Verification items for the finished model (mm, model axes). Face numbers are marked on the shaded views. A direction names the side the tool comes from. Round coordinates to 2 decimals unless told otherwise and drop trailing zeros. Write each loop counter-clockwise with the first axis right and the second up, starting at its lowest first coordinate (ties: lowest second). Pieces come first, ordered by that corner, then holes. Notation, with made-up numbers: (14, 29) - (20, 29) arc R19 ccw to (20, 33) - close; hole circle Ø6 at (-29.75, 68.25). An arc over 180 degrees is marked (long way). Answer as a JSON object with one key per item and string values.
```python
from build123d import *

# Parameters (mm, degrees)
CROQUIS1_W              = 54
CROQUIS1_H              = 41
CROQUIS1_R              = 3.75
SALIENTE_EXTRUIR1_DEPTH = 24
CROQUIS2_W              = 32
CROQUIS2_H              = 41
CORTAR_EXTRUIR1_DEPTH   = 16
CROQUIS3_R              = 2.5
CORTAR_EXTRUIR2_DEPTH   = 63.547981582
CHAFL_N1_SIZE           = 4
CORTAR_EXTRUIR3_REACH   = 43.536
CROQUIS4_R              = 10


with BuildPart() as part:
    # Croquis1 → Saliente-Extruir1 (new body)
    with BuildSketch(Plane.XY):
        Rectangle(CROQUIS1_W, CROQUIS1_H)
        with Locations((-21.5, 7.5)):
            Circle(CROQUIS1_R, mode=Mode.SUBTRACT)
        with Locations((21.5, 7.5)):
            Circle(CROQUIS1_R, mode=Mode.SUBTRACT)
        with Locations((21.5, -14.5)):
            Circle(CROQUIS1_R, mode=Mode.SUBTRACT)
        with Locations((-21.5, -14.5)):
            Circle(CROQUIS1_R, mode=Mode.SUBTRACT)
    extrude(amount=-SALIENTE_EXTRUIR1_DEPTH)

    # Croquis2 → Cortar-Extruir1 (cut)
    with BuildSketch(Plane(origin=(0, 0, -24), x_dir=(-1, 0, 0), z_dir=(0, 0, -1))):
        Rectangle(CROQUIS2_W, CROQUIS2_H)
    extrude(amount=-CORTAR_EXTRUIR1_DEPTH, mode=Mode.SUBTRACT)

    # Croquis3 → Cortar-Extruir2 (cut, through all)
    with BuildSketch(Plane(origin=(27, 0, 0), x_dir=(0, 0, -1), z_dir=(1, 0, 0))):
        with Locations(Location((17, 15.5, 0), (0, 0, 90))):
            Circle(CROQUIS3_R)
    extrude(amount=-CORTAR_EXTRUIR2_DEPTH, mode=Mode.SUBTRACT)

    # Chaflán1
    chafl_n1_edges = [part.edges().sort_by_distance(p)[0] for p in [
        (0, 20.5, 0),
    ]]
    chamfer(chafl_n1_edges, length=CHAFL_N1_SIZE)

    # Croquis4 → Cortar-Extruir3 (cut, up to next)
    with BuildSketch(Plane.XY, mode=Mode.PRIVATE) as cortar_extruir3_sk1:
        with Locations((0, -2.5)):
            Circle(CROQUIS4_R)
    cortar_extruir3_tool1 = extrude(cortar_extruir3_sk1.sketch, amount=-CORTAR_EXTRUIR3_REACH, mode=Mode.PRIVATE) & part.part
    add(cortar_extruir3_tool1.solids().sort_by_distance((0, -2.5, 0))[0], mode=Mode.SUBTRACT)


solid = part.part
```
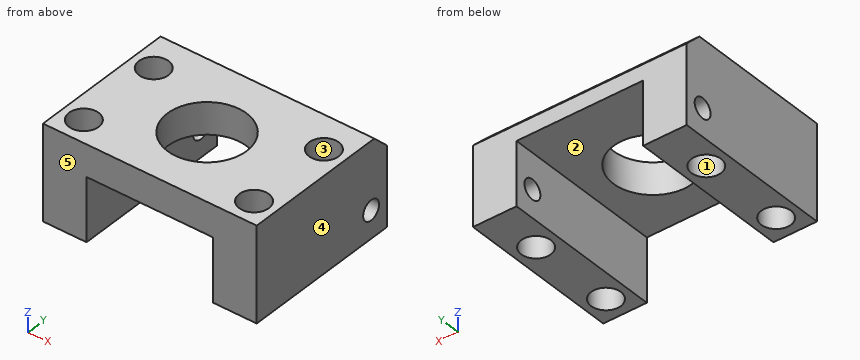
Q1. Material ranges on line 1 along Y through (x, z) = (21.5, -13.25); line 2 along X through (y, z) = (-6, -12); line 3 along Y through (x, z) = (0, -4), recorded low to high. Write a range as [from, to].
Geometry check:
{"line 1": "y = [-20.5, -18.25], [-10.75, 3.75], [11.25, 20.5]", "line 2": "x = [-27, -16], [16, 27]", "line 3": "y = [-20.5, -12.5], [7.5, 20.5]"}
Q2. Gauge pin test, flat ends, axial feed: P1, Ø1, axis at x = -11.5, y = 7, coming from the -Z side; P2, Ø7, axis at x = -21.5, y = -14.5, coming from the -Z side; P3, Ø23, axis at x = 0, y = -2.5, coming from the +Z side. Record the tip position at first contact, or that the pin passes through.
Geometry check:
{"P1": "stops at z = -8", "P2": "passes through", "P3": "stops at z = 0"}
Q3. Set-up check for the marked faces 1 and 2: record each of +Z, -Z, +X, -X, +Y, -Y from which the full face is reachable in a straight line by a thin tool's end or side.
Geometry check:
{"face 1": "+Z, -Z", "face 2": "-Z, +Y, -Y"}
Q4. Section check B-B, the plane z = -13.5. Record the cut outline in (x, y), then the cut area to 3 significant figures.
Geometry check:
{"outline": "(-27, -20.5) - (-16, -20.5) - (-16, 20.5) - (-27, 20.5) - close; (16, -20.5) - (27, -20.5) - (27, 20.5) - (16, 20.5) - close; hole circle Ø7.5 at (-21.5, -14.5); hole circle Ø7.5 at (-21.5, 7.5); hole circle Ø7.5 at (21.5, -14.5); hole circle Ø7.5 at (21.5, 7.5)", "area": "725 mm2"}
Q5. Release check for a two-part mould opening along X. For the marked faces 3, 4 and 5 record: released by +X, released by -X, zero draft, split by the parting line, or undercut.
Geometry check:
{"face 3": "undercut", "face 4": "released by +X", "face 5": "zero draft"}
Q6. Section check A-A, the plane x = -21.5. Record the cut outline in (y, z).
Geometry check:
{"outline": "(-20.5, -24) - (-18.25, -24) - (-18.25, 0) - (-20.5, 0) - close; (-10.75, -24) - (3.75, -24) - (3.75, 0) - (-10.75, 0) - close; (11.25, -24) - (20.5, -24) - (20.5, -4) - (16.5, 0) - (11.25, 0) - close; hole circle Ø5 at (15.5, -17)"}
Q7. Section check C-C, the plane y = -2.5. Record the cut outline in (x, z).
Geometry check:
{"outline": "(-27, -24) - (-16, -24) - (-16, -8) - (-10, -8) - (-10, 0) - (-27, 0) - close; (10, -8) - (16, -8) - (16, -24) - (27, -24) - (27, 0) - (10, 0) - close"}
Q8. Section check D-D, the plane x = 0. Record the cut outline in (y, z).
Geometry check:
{"outline": "(-20.5, -8) - (-12.5, -8) - (-12.5, 0) - (-20.5, 0) - close; (7.5, -8) - (20.5, -8) - (20.5, -4) - (16.5, 0) - (7.5, 0) - close"}
